from build123d import *

# Parameters (mm, degrees)
F0_W     = 40
F0_H     = 40
F1_DEPTH = 3
F2_R     = 5
F3_DEPTH = 40
F4_R     = 15
F5_DEPTH = 30
F6_R     = 15
F7_R     = 5


with BuildPart() as f1:
    # F0 (on Top) → F1 (new body)
    with BuildSketch(Plane.XY):
        Rectangle(F0_W, F0_H)
    extrude(amount=F1_DEPTH)

    # F2 (on face) → F3 (join)
    with BuildSketch(Plane.XY.offset(3)):
        Circle(F2_R)
    extrude(amount=F3_DEPTH)

    # F4 (on face) → F5 (join)
    with BuildSketch(Plane.XY.offset(43)):
        Circle(F4_R)
    extrude(amount=F5_DEPTH)

    # F6
    f6_edges = [f1.edges().sort_by_distance(p)[0] for p in [
        (-15, 0, 73),
    ]]
    fillet(f6_edges, radius=F6_R)

    # F7
    f7_edges = [f1.edges().sort_by_distance(p)[0] for p in [
        (-15, 0, 43),
    ]]
    fillet(f7_edges, radius=F7_R)


solid = f1.part
CAD build for the part. Positions are in the model's coordinates, mm. A direction names the side the tool comes from. Round coordinates to 2 decimals unless told otherwise and drop trailing zeros. Write each loop counter-clockwise with the first axis right and the second up, starting at its lowest first coordinate (ties: lowest second). Pieces come first, ordered by that corner, then holes.
(1) Slice it at D-D, the plane y = -17. Write the cut outline in (x, z), and give its area (3 significant figures).
(2) Probe line 1 along Z through (x, y) = (-15, -2); line 2 along Z through (x, y) = (-7, -11.5); line 3 along Z through (x, y) = (-1, 8). List the from-to ranges inside material, lowest first.
(3) 3-axis set-ups, long thin cutter, end or side, ignore diameter. For faces 1 (the face through (20, 0, 1)), 2 (the face through (-1.08, -4.88, 22.72)), 3 (the face through (-14.985, 0.66, 52.93)): which of +Z, -Z, +X, -X, +Y, -Y reach the whole face in a straight line?
(4) Slice it at C-C, the plane z = 36. Write the cut outline in (x, y).
(5) Drop flat-ended pins along their axis: P1, Ø8, axis at y = 10, z = 17, coming from the -X side; P2, Ø1.5, axis at y = -5, z = 39, coming from the -X side; P3, Ø2, axis at y = 5, z = 58.5, coming from the -X side; P4, Ø1, axis at x = -7.5, z = 52, coming from the -Y side. Give the stop position or say it passes through.
(6) Slice it at A-A, the plane x = 0. Write the cut outline in (y, z), and give its area (3 significant figures).
From the geometry:
1. outline: (-20, 0) - (20, 0) - (20, 3) - (-20, 3) - close
1. area: 120 mm2
2. line 1: z = 0 to 3
2. line 2: z = 0 to 3, 44.39 to 64.61
2. line 3: z = 0 to 3, 43 to 70.65
3. face 1: +Z, -Z, +X, +Y, -Y
3. face 2: none
3. face 3: +Z
4. outline: circle Ø10 at (0, 0)
5. P1: passes through
5. P2: stops at x = -2.63
5. P3: stops at x = -14.45
5. P4: stops at y = -13.27
6. outline: (-20, 0) - (20, 0) - (20, 3) - (5, 3) - (5, 43) - (10, 43) arc R5 ccw to (15, 48) - (15, 58) arc R15 ccw to (-15, 58) - (-15, 48) arc R5 ccw to (-10, 43) - (-5, 43) - (-5, 3) - (-20, 3) - close
6. area: 1,310 mm2
